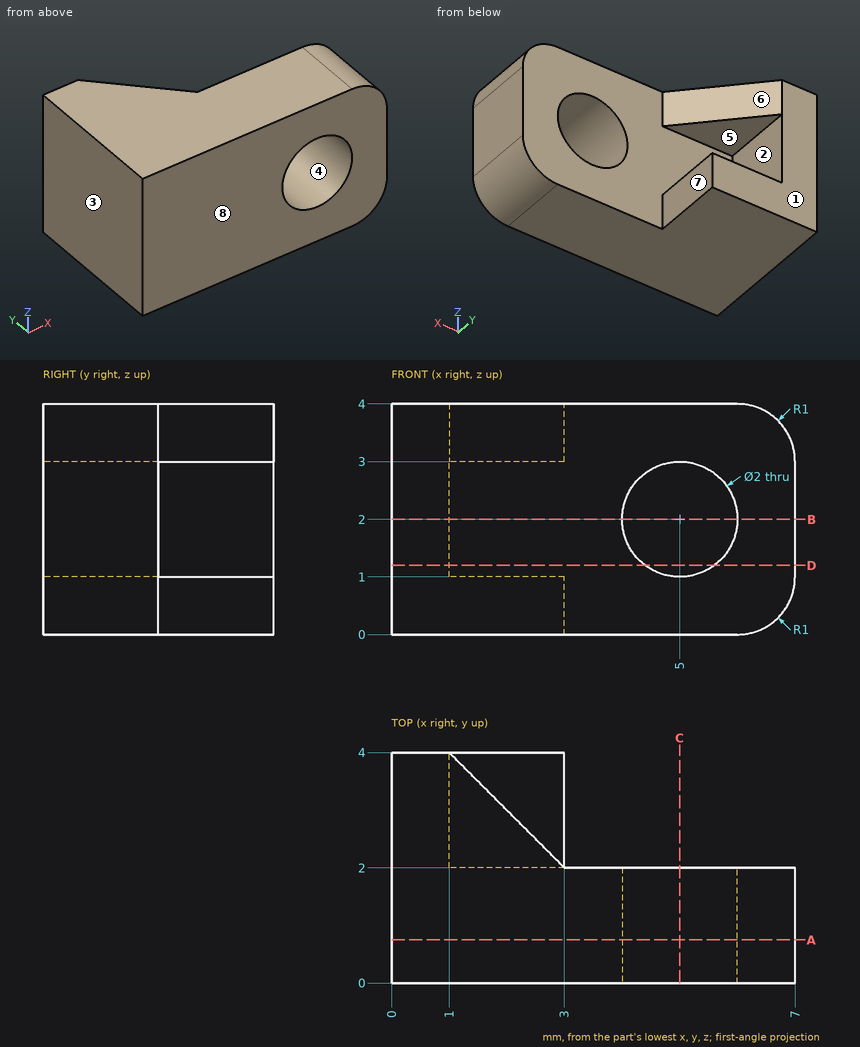
Geometry check sheet. Reference: drawing and pictorial views, mm from the part's lowest x, y, z. A direction names the side the tool comes from. Give positions to 0.01 mm unless a question says otherwise; leave off trailing zeros. Write each loop counter-clockwise with the first axis right and the second up, starting at its lowest first coordinate (ties: lowest second). Pieces come first, ordered by that corner, then holes.
Item 1: Cross-section at A-A (y = 0.75). Enter the section's corners in (x, z), and give its area (3 significant figures).
Item 2: Scan lines: L1, parallel to Z at x = 5, y = 1.2; L2, parallel to X at y = 0.75, z = 2; L3, parallel to Y at x = 4, z = 3.1. Record each from-to range of solid material in increasing order.
Item 3: Cross-section at C-C (x = 5). Enter the section's corners in (y, z), and give its area (3 significant figures).
Item 4: Cross-section at D-D (z = 1.2). Enter the section's corners in (x, y), and give its area (3 significant figures).
Item 5: Cross-section at B-B (z = 2). Enter the section's corners in (x, y).
Item 6: Access from +Z, -Z, +X, -X, +Y, -Y to the whole of each face (thin tool, end or side, straight path). Record for the marked faces 5, 6, 7 and 8.
Item 7: Gauge pin test, flat ends, axial feed: pin 1 (0.8 mm diameter, centred on y = 2.5, z = 0.5, fed in from +X); pin 2 (0.6 mm diameter, centred on y = 3, z = 2.5, fed in from +X); pin 3 (1.2 mm diameter, centred on x = 3, z = 2, fed in from +Y). Record the tip position at first contact, or that the pin passes through.
Item 8: Draft check along X on the marked faces 1, 2, 3 and 4. Enter one of: released by +X, released by -X, zero draft, split by the parting line, or undercut.
Report:
1. outline: (0, 0) - (6, 0) arc R1 ccw to (7, 1) - (7, 3) arc R1 ccw to (6, 4) - (0, 4) - close; hole circle Ø2 at (5, 2)
1. area: 24.4 mm2
2. L1: z = 0 to 1, 3 to 4
2. L2: x = 0 to 4, 6 to 7
2. L3: y = 0 to 2
3. outline: (0, 0) - (2, 0) - (2, 1) - (0, 1) - close; (0, 3) - (2, 3) - (2, 4) - (0, 4) - close
3. area: 4.00 mm2
4. outline: (0, 0) - (4.4, 0) - (4.4, 2) - (1, 2) - (1, 4) - (0, 4) - close; (5.6, 0) - (7, 0) - (7, 2) - (5.6, 2) - close
4. area: 13.6 mm2
5. outline: (0, 0) - (4, 0) - (4, 2) - (1, 2) - (1, 4) - (0, 4) - close; (6, 0) - (7, 0) - (7, 2) - (6, 2) - close
6. face 5: +X, +Y
6. face 6: +Z, +X, +Y
6. face 7: +Z, -Z, +X, +Y
6. face 8: +Z, -Z, +X, -X, -Y
7. pin 1: stops at x = 3
7. pin 2: stops at x = 1
7. pin 3: stops at y = 2
8. face 1: zero draft
8. face 2: released by +X
8. face 3: released by -X
8. face 4: undercut
